The listing builds one solid part. Answer for the finished solid, in the listing's coordinates (mm). A direction names the side the tool comes from. Give positions to 0.01 mm unless a question says otherwise; leave off trailing zeros. Loops run counter-clockwise (first coordinate to the right, second up) from the corner with the lowest first, then second, coordinate; pieces in that order, holes last. Notation, with made-up numbers: (48, 77.25) - (59, 77.25) arc R22 ccw to (59, 93.25) - close; hole circle Ø4 at (-12.5, -7.75). An arc over 180 degrees is marked (long way). Write item = value, one per line. Start each with the question number.
1) Consider probe 1 along X at (y, z) = (31.5, -12.2); probe 2 along Z at (x, y) = (-12.2, 45.5); probe 3 along X at (y, z) = (70.5, -24.7). Determine where each line is inside the solid, lowest interval first.
2) The mould has two halves that part along X. Classify faces 1 (the flat face through (26, 2, -15.7)), 2 (the cylindrical face through (-26.917, 2.532, 26.847)), 3 (the flat face through (8.7, 2, 26)), 4 (the cylindrical face through (-13.465, 56.737, -23.894)): +X half, -X half, draft (parallel to the pull), parting line (faces both ways), or undercut.
3) Which of the six approach directions +Z, -Z, +X, -X, +Y, -Y give full straight-line access (tool end or side, diameter ignored) to faces 5 (the cylindrical face through (25.5, 2.5, 25.3)), 6 (the flat face through (-26, 3, 11)), 7 (the cylindrical face through (-6, 110, 0)), 8 (the flat face through (26, 3, -11))?
4) The part is cut by section A-A on y = 73. Write down the section's boundary in (x, z), plus the area to 3 significant figures.
5) Flat-ended cylindrical pins translate along their axes: P1, Ø3, axis at x = 26.5, y = 1.5, coming from the -Z side; P2, Ø1.6, axis at y = 69, z = 25.5, coming from the -X side; P3, Ø0.9, axis at x = 25.5, y = 64, coming from the +Z side. Find the tip coordinate at first contact, or state that the pin passes through.
from build123d import *

# Parameters (mm, degrees)
SKETCH_R              = 19.05
PAD_DEPTH             = 1.6
SKETCH001_W           = 56.4
SKETCH001_H           = 56.4
PAD001_DEPTH          = 112
SKETCH002_R           = 6
POCKET_DEPTH          = 2.5
SKETCH003_R           = 3.175
PAD002_DEPTH          = 21.9
SKETCH004_R           = 6
POCKET001_DEPTH       = 4
SKETCH005_W           = 9.13
SKETCH005_H           = 9.13
POCKET002_DEPTH       = 1000
POLARPATTERN_COUNT    = 4
SKETCH006_R           = 2.5
POCKET003_DEPTH       = 5
POLARPATTERN001_COUNT = 4
POCKET004_DEPTH       = 3
POLARPATTERN002_COUNT = 4
FILLET_R              = 4.5
FILLET001_R           = 1.5
SKETCH008_R           = 1.5
POCKET005_DEPTH       = 1000
POLARPATTERN003_COUNT = 4
CHAMFER_SIZE          = 0.5
CHAMFER001_SIZE       = 0.2


with BuildPart() as part:
    # Sketch → Pad (new body)
    with BuildSketch(Plane.XZ):
        Circle(SKETCH_R)
    extrude(amount=PAD_DEPTH)

    # Sketch001 (on Face2 of Pad) → Pad001 (join)
    with BuildSketch(Plane(origin=(0, 0, 0), x_dir=(1, 0, 0), z_dir=(0, 1, 0))):
        Rectangle(SKETCH001_W, SKETCH001_H)
    extrude(amount=PAD001_DEPTH)

    # Sketch002 (on Face8 of Pad001) → Pocket (cut)
    with BuildSketch(Plane.XZ.offset(1.6)):
        Circle(SKETCH002_R)
    extrude(amount=-POCKET_DEPTH, mode=Mode.SUBTRACT)

    # Sketch003 (on Face10 of Pocket) → Pad002 (join)
    with BuildSketch(Plane.XZ.offset(-0.9)):
        Circle(SKETCH003_R)
    extrude(amount=PAD002_DEPTH)

    # Sketch004 (on Face5 of Pad002) → Pocket001 (cut)
    with BuildSketch(Plane(origin=(0, 112, 0), x_dir=(1, 0, 0), z_dir=(0, 1, 0))):
        Circle(SKETCH004_R)
    extrude(amount=-POCKET001_DEPTH, mode=Mode.SUBTRACT)

    # Sketch005 (on DatumPlane) → Pocket002 (cut)
    with BuildSketch(Plane.XZ.offset(-5)):
        with Locations((-23.635, 23.635)):
            Rectangle(SKETCH005_W, SKETCH005_H)
    pocket002 = extrude(amount=-POCKET002_DEPTH, mode=Mode.SUBTRACT)

    # PolarPattern: Pocket002 ×4 about axis
    polarpattern_axis = Axis((0, 5, 0), (0, -1, 0))
    for i in range(1, POLARPATTERN_COUNT):
        add(pocket002.rotate(polarpattern_axis, i * 360 / POLARPATTERN_COUNT), mode=Mode.SUBTRACT)

    # Sketch006 (on Face12 of PolarPattern) → Pocket003 (cut)
    with BuildSketch(Plane(origin=(0, 5, 0), x_dir=(1, 0, 0), z_dir=(0, 1, 0))):
        with Locations((-23.635, 23.635)):
            Circle(SKETCH006_R)
    pocket003 = extrude(amount=-POCKET003_DEPTH, mode=Mode.SUBTRACT)

    # PolarPattern001: Pocket003 ×4 about axis
    polarpattern001_axis = Axis((0, 5, 0), (0, 1, 0))
    for i in range(1, POLARPATTERN001_COUNT):
        add(pocket003.rotate(polarpattern001_axis, i * 360 / POLARPATTERN001_COUNT), mode=Mode.SUBTRACT)

    # Sketch007 (on Face2 of Pocket003) → Pocket004 (cut)
    with BuildSketch(Plane.XZ):
        with BuildLine():
            ThreePointArc((-15.7, -33.555168), (-12.2, -37.055168), (-8.7, -33.555168))
            Line((-8.7, -33.555168), (-8.7, -24.7))
            ThreePointArc((-8.7, -24.7), (-12.2, -21.2), (-15.7, -24.7))
            Line((-15.7, -33.555168), (-15.7, -24.7))
        make_face()
    pocket004 = extrude(amount=-POCKET004_DEPTH, mode=Mode.SUBTRACT)

    # PolarPattern002: Pocket004 ×4 about axis
    polarpattern002_axis = Axis((0, 0, 0), (0, -1, 0))
    for i in range(1, POLARPATTERN002_COUNT):
        add(pocket004.rotate(polarpattern002_axis, i * 360 / POLARPATTERN002_COUNT), mode=Mode.SUBTRACT)

    # Fillet
    fillet_edges = [part.edges().sort_by_distance(p)[0] for p in [
        (-19.07, 58.5, -19.07),
        (-28.2, 2.5, -28.2),
        (-19.07, 58.5, 19.07),
        (-28.2, 2.5, 28.2),
        (19.07, 58.5, 19.07),
        (28.2, 2.5, 28.2),
        (19.07, 58.5, -19.07),
        (28.2, 2.5, -28.2),
    ]]
    fillet(fillet_edges, radius=FILLET_R)

    # Fillet001
    fillet001_edges = [part.edges().sort_by_distance(p)[0] for p in [
        (28.2, 58.5, 19.07),
        (19.07, 58.5, 28.2),
        (-19.07, 58.5, 28.2),
        (-28.2, 58.5, 19.07),
        (-28.2, 58.5, -19.07),
        (-19.07, 58.5, -28.2),
        (28.2, 58.5, -19.07),
        (19.07, 58.5, -28.2),
    ]]
    fillet(fillet001_edges, radius=FILLET001_R)

    # Sketch008 (on Face12 of Fillet001) → Pocket005 (cut)
    with BuildSketch(Plane.XZ.offset(-3)):
        with Locations((-24.7, 12.2)):
            Circle(SKETCH008_R)
    pocket005 = extrude(amount=-POCKET005_DEPTH, mode=Mode.SUBTRACT)

    # PolarPattern003: Pocket005 ×4 about axis
    polarpattern003_axis = Axis((0, 3, 0), (0, -1, 0))
    for i in range(1, POLARPATTERN003_COUNT):
        add(pocket005.rotate(polarpattern003_axis, i * 360 / POLARPATTERN003_COUNT), mode=Mode.SUBTRACT)

    # Chamfer
    chamfer_edges = [part.edges().sort_by_distance(p)[0] for p in [
        (-3.175, -21, 0),
    ]]
    chamfer(chamfer_edges, length=CHAMFER_SIZE)

    # Chamfer001
    chamfer001_edges = [part.edges().sort_by_distance(p)[0] for p in [
        (-26.881981, 0, 26.881981),
        (-28.2, 0, -7.5),
        (7.5, 0, -28.2),
        (28.2, 0, 7.5),
        (-19.05, 0, 0),
        (-19.05, -1.6, 0),
        (-6, -1.6, 0),
        (-28.2, 1.5, 8.7),
        (-28.2, 3, 12.2),
        (-28.2, 1.5, 15.7),
        (-15.7, 1.5, -28.2),
        (-12.2, 3, -28.2),
        (-8.7, 1.5, -28.2),
        (28.2, 1.5, -15.7),
        (28.2, 3, -12.2),
        (28.2, 1.5, -8.7),
        (15.7, 1.5, 28.2),
        (12.2, 3, 28.2),
        (8.7, 1.5, 28.2),
        (-21.2, 0, 12.2),
        (-12.2, 0, -21.2),
        (21.2, 0, -12.2),
        (12.2, 0, 21.2),
        (-20.388019, 112, 20.388019),
        (-26.881981, 5, 26.881981),
        (26.881981, 5, 26.881981),
        (-26.881981, 5, -26.881981),
        (26.881981, 5, -26.881981),
        (-6, 112, 0),
    ]]
    chamfer(chamfer001_edges, length=CHAMFER001_SIZE)


solid = part.part
Answer below:
q1.probe_1 = -28.2 to 23.2, 26.2 to 28.2
q1.probe_2 = -28.2 to -26.2, -23.2 to 28.2
q1.probe_3 = -19.07 to -13.7, -10.7 to 19.07
q2.face_1 = draft
q2.face_2 = -X half
q2.face_3 = undercut
q2.face_4 = undercut
q3.face_5 = +Y, -Y
q3.face_6 = -X, -Y
q3.face_7 = +Y
q3.face_8 = +X, -Y
q4.outline = (-28.2, -17.57) arc R1.5 ccw to (-26.7, -19.07) - (-23.57, -19.07) arc R4.5 cw to (-19.07, -23.57) - (-19.07, -26.7) arc R1.5 ccw to (-17.57, -28.2) - (17.57, -28.2) arc R1.5 ccw to (19.07, -26.7) - (19.07, -23.57) arc R4.5 cw to (23.57, -19.07) - (26.7, -19.07) arc R1.5 ccw to (28.2, -17.57) - (28.2, 17.57) arc R1.5 ccw to (26.7, 19.07) - (23.57, 19.07) arc R4.5 cw to (19.07, 23.57) - (19.07, 26.7) arc R1.5 ccw to (17.57, 28.2) - (-17.57, 28.2) arc R1.5 ccw to (-19.07, 26.7) - (-19.07, 23.57) arc R4.5 cw to (-23.57, 19.07) - (-26.7, 19.07) arc R1.5 ccw to (-28.2, 17.57) - close; hole circle Ø3 at (-24.7, 12.2); hole circle Ø3 at (-12.2, -24.7); hole circle Ø3 at (12.2, 24.7); hole circle Ø3 at (24.7, -12.2)
q4.area = 2,830 mm2
q5.P1 = -28.01
q5.P2 = -19.07
q5.P3 = 19.07
